Source: CAD feature listing. Evaluate the final solid. Frame: model axes, mm. A direction names the side the tool comes from. Give positions to 0.01 mm unless a question says otherwise; leave off trailing zeros. Write each loop counter-clockwise with the first axis right and the second up, starting at its lowest first coordinate (ties: lowest second). Pieces come first, ordered by that corner, then holes. Notation, with made-up numbers: (-38.5, -22.75) -> (-29.5, -22.75) arc R25 cw to (-29.5, -8.75) -> close; hole circle Ø7 at (-4, 40.25). An arc over 180 degrees is marked (long way). Use one line per item in the form item = value. Start each with the question number.
(1) Cut plane C-C, the plane y = 0.9. Output: boundary loops of the cut face in (x, z), and give its area (3 significant figures).
(2) Cut plane B-B, the plane x = 25. Output: boundary loops of the cut face in (y, z).
(3) Draft query along X for faces 5 (the face through (19.1, 1.52, -0.86)), 6 (the face through (-17, 2, -20)), 7 (the face through (0.86, 1.52, -0.9)), 8 (the face through (-30.68, 1.52, -31.08)). Return one class per face: pulls with the +X half, pulls with the -X half, needs draft (parallel to the pull), parting line crosses it, or undercut.
(4) Cut plane A-A, the plane z = -30. Output: boundary loops of the cut face in (x, y).
(5) Set-up query: faces 1 (the face through (4, 0, -30)), 2 (the face through (20, 1, -50)), 3 (the face through (20, 1, -10)), 4 (the face through (0, 1, -50)). Return all of +Z, -Z, +X, -X, +Y, -Y with unobstructed straight access to the full face (end or side cutting, diameter ignored); none if empty.
(6) Material intervals for line 1 along Z through (x, y) = (10, 1.45); line 2 along X through (y, z) = (2.45, -30); line 3 along Z through (x, y) = (25, 0.75), sorted ascending. Write a range as from..to.
(7) Cut plane D-D, the plane z = -7. Output: boundary loops of the cut face in (x, y), and give its area (3 significant figures).
(8) First-contact query: P1, Ø0.9, axis at y = 1, z = -50, coming from the +X side; P2, Ø1.5, axis at x = -15, y = 1, coming from the -Z side; P3, Ø1.5, axis at y = 1.5, z = -8.5, coming from the -X side. Flat tips, straight axial feed; report the tip coordinate or a pass-through.
from build123d import *

# Parameters (mm, degrees)
SKETCH_1_W      = 20
SKETCH_1_H      = 60
SKETCH_1_R      = 2.6
EXTRUDE_1_DEPTH = 3
SKETCH_2_W      = 34.5
SKETCH_2_H      = 20
SKETCH_2_R      = 1.6
SKETCH_2_W_2    = 10
EXTRUDE_2_DEPTH = 3
FILLET_1_R      = 3


with BuildPart() as part:
    # 草图1 → 凸台-拉伸1 (new body)
    with BuildSketch(Plane(origin=(0, 0, 0), x_dir=(1, 0, 0), z_dir=(0, 1, 0))):
        with Locations((10, 30)):
            Rectangle(SKETCH_1_W, SKETCH_1_H)
        with Locations((10, 7)):
            Circle(SKETCH_1_R, mode=Mode.SUBTRACT)
        with Locations((10, 53)):
            Circle(SKETCH_1_R, mode=Mode.SUBTRACT)
    extrude(amount=EXTRUDE_1_DEPTH)

    # 草图2 → 凸台-拉伸2 (add)
    with BuildSketch(Plane(origin=(0, 3, 0), x_dir=(1, 0, 0), z_dir=(0, 1, 0))):
        with Locations((-17.25, 30)):
            Rectangle(SKETCH_2_W, SKETCH_2_H)
        with Locations((-29.5, 30)):
            Circle(SKETCH_2_R, mode=Mode.SUBTRACT)
        with Locations((25, 30)):
            Rectangle(SKETCH_2_W_2, SKETCH_2_H)
        with Locations((25, 30)):
            Circle(SKETCH_2_R, mode=Mode.SUBTRACT)
    extrude(amount=-EXTRUDE_2_DEPTH)

    # 圆角1
    fillet_1_edges = [part.edges().sort_by_distance(p)[0] for p in [
        (0, 1.5, -40),
        (0, 1.5, -20),
        (-34.5, 1.5, -20),
        (-34.5, 1.5, -40),
        (20, 1.5, -20),
        (20, 1.5, -40),
        (30, 1.5, -40),
        (30, 1.5, -20),
        (0, 1.5, -60),
        (20, 1.5, -60),
        (20, 1.5, 0),
        (0, 1.5, 0),
    ]]
    fillet(fillet_1_edges, radius=FILLET_1_R)


solid = part.part
Geometry says:
q1.outline = (-34.5, -37) arc R3 ccw to (-31.5, -40) -> (-3, -40) arc R3 cw to (0, -43) -> (0, -57) arc R3 ccw to (3, -60) -> (17, -60) arc R3 ccw to (20, -57) -> (20, -43) arc R3 cw to (23, -40) -> (27, -40) arc R3 ccw to (30, -37) -> (30, -23) arc R3 ccw to (27, -20) -> (23, -20) arc R3 cw to (20, -17) -> (20, -3) arc R3 ccw to (17, 0) -> (3, 0) arc R3 ccw to (0, -3) -> (0, -17) arc R3 cw to (-3, -20) -> (-31.5, -20) arc R3 ccw to (-34.5, -23) -> close; hole circle Ø3.2 at (-29.5, -30); hole circle Ø5.2 at (10, -53); hole circle Ø5.2 at (10, -7); hole circle Ø3.2 at (25, -30)
q1.area = 2,020 mm^2
q2.outline = (0, -40) -> (3, -40) -> (3, -31.6) -> (0, -31.6) -> close; (0, -28.4) -> (3, -28.4) -> (3, -20) -> (0, -20) -> close
q3.face_5 = pulls with the +X half
q3.face_6 = needs draft
q3.face_7 = pulls with the -X half
q3.face_8 = undercut
q4.outline = (-34.5, 0) -> (-31.1, 0) -> (-31.1, 3) -> (-34.5, 3) -> close; (-27.9, 0) -> (23.4, 0) -> (23.4, 3) -> (-27.9, 3) -> close; (26.6, 0) -> (30, 0) -> (30, 3) -> (26.6, 3) -> close
q5.face_1 = +Z, -Z, +X, -X, -Y
q5.face_2 = -Z, +X, +Y, -Y
q5.face_3 = +Z, +X, +Y, -Y
q5.face_4 = -Z, -X, +Y, -Y
q6.line_1 = -60..-55.6, -50.4..-9.6, -4.4..0
q6.line_2 = -34.5..-31.1, -27.9..23.4, 26.6..30
q6.line_3 = -40..-31.6, -28.4..-20
q7.outline = (0, 0) -> (7.4, 0) -> (7.4, 3) -> (0, 3) -> close; (12.6, 0) -> (20, 0) -> (20, 3) -> (12.6, 3) -> close
q7.area = 44.4 mm^2
q8.P1 = 20
q8.P2 = -40
q8.P3 = 0
